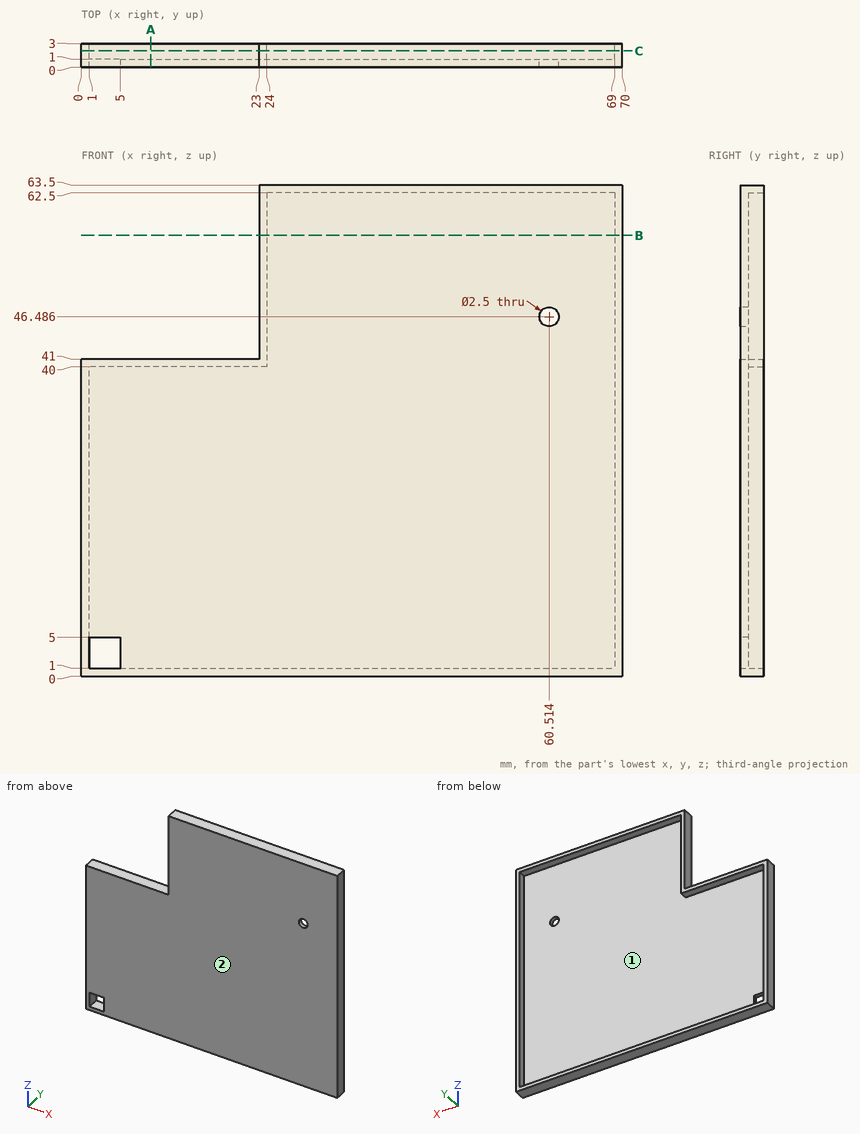
Geometry check sheet. Reference: drawing and pictorial views, mm from the part's lowest x, y, z. Give positions to 0.01 mm unless a question says otherwise; leave off trailing zeros. Loops run counter-clockwise (first coordinate to the right, second up) from the corner with the lowest first, then second, coordinate; pieces in that order, holes last.
1. Section check B-B, the plane z = 57. Enter the section's corners in (x, y), then the cut area to 3 significant figures.
2. Go/stop test with flat-tipped pins: pin 1 Ø3 at (x, z) = (60.51, 46.49) entering from +Y; pin 2 Ø0.9 at (x, y) = (16.5, 1) entering from +Z. Record where each tip stops, or that it passes through.
3. Mould release check, pull along Z, two halves, no side actions. Record for the marked faces 1 and 2: released by +Z, released by -Z, zero draft, split by the parting line, or undercut.
4. Section check C-C, the plane y = 2.1. Enter the section's corners in (x, z).
5. Thickness scan on line 1 (Z direction, x = 18.5, y = 1.7); line 2 (X direction, y = 2.45, z = 57.5); line 3 (Z direction, x = 37.5, y = 1.5). Record the ranges inside material, lowest first.
6. Section check A-A, the plane x = 9. Enter the section's corners in (y, z), then the cut area to 3 significant figures.
Geometry says:
1. outline: (23, 0) - (70, 0) - (70, 3) - (69, 3) - (69, 1) - (24, 1) - (24, 3) - (23, 3) - close
1. area: 51.0 mm2
2. pin 1: stops at y = 1
2. pin 2: stops at z = 41
3. face 1: undercut
3. face 2: zero draft
4. outline: (0, 0) - (70, 0) - (70, 63.5) - (23, 63.5) - (23, 41) - (0, 41) - close; hole (1, 1) - (69, 1) - (69, 62.5) - (24, 62.5) - (24, 40) - (1, 40) - close
5. line 1: z = 0 to 1, 40 to 41
5. line 2: x = 23 to 24, 69 to 70
5. line 3: z = 0 to 1, 62.5 to 63.5
6. outline: (0, 0) - (3, 0) - (3, 1) - (1, 1) - (1, 40) - (3, 40) - (3, 41) - (0, 41) - close
6. area: 45.0 mm2
